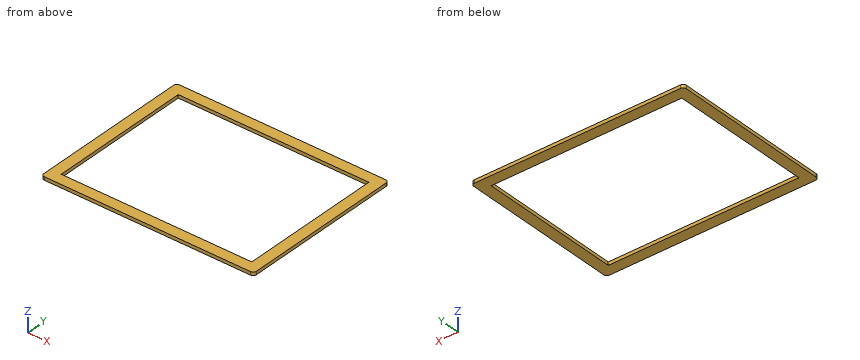
```python
from build123d import *

# Parameters (mm, degrees)
F0_W     = 194
F0_H     = 150
F1_DEPTH = 3
F2_W     = 174
F2_H     = 130
F3_DEPTH = 3
F4_R     = 3


with BuildPart() as f1:
    # F0 (on Top) → F1 (new body)
    with BuildSketch(Plane.XY):
        Rectangle(F0_W, F0_H)
    extrude(amount=F1_DEPTH)

    # F2 (on face) → F3 (cut, through all)
    with BuildSketch(Plane.XY.offset(3)):
        Rectangle(F2_W, F2_H)
    extrude(amount=-F3_DEPTH, mode=Mode.SUBTRACT)

    # F4
    f4_edges = [f1.edges().sort_by_distance(p)[0] for p in [
        (-97, -75, 1.5),
        (97, -75, 1.5),
        (97, 75, 1.5),
        (-97, 75, 1.5),
    ]]
    fillet(f4_edges, radius=F4_R)


solid = f1.part
```
Model file for the job. Use its own axes, mm. Coordinates: 2 decimals unless noted, no trailing zeros. Order: outer loops, then holes, each group sorted by start corner. A loop starts at its lowest first (then second) coordinate and runs counter-clockwise, first axis right, second up. Notation, with made-up numbers: M 40,-23.75 L 71,-23.75 A15 cw 71,-0.75 Z; hole C 85,-23 d8. An arc over 180 degrees is marked long. Answer as CSV lines item,"result".
(1) Band-saw the part on B-B, the plane z = 0.9. List the corners of the cut face in (x, y), then the cut area to 3 significant figures.
Geometry says:
outline,"M -97,-72 A3 ccw -94,-75 L 94,-75 A3 ccw 97,-72 L 97,72 A3 ccw 94,75 L -94,75 A3 ccw -97,72 Z; hole M -87,-65 L 87,-65 L 87,65 L -87,65 Z"
area,"6,470 mm2"
(2) Band-saw the part on C-C, the plane y = -29.5. List the corners of the cut face in (x, z).
Geometry says:
outline,"M -97,0 L -87,0 L -87,3 L -97,3 Z; M 87,0 L 97,0 L 97,3 L 87,3 Z"
(3) Band-saw the part on A-A, the plane x = -84.5. List the corners of the cut face in (y, z), then the cut area to 3 significant figures.
Geometry says:
outline,"M -75,0 L -65,0 L -65,3 L -75,3 Z; M 65,0 L 75,0 L 75,3 L 65,3 Z"
area,"60.0 mm2"
(4) Wall check: line 1 along X through (y, z) = (-26, 2.8); line 2 along Y through (x, z) = (72.5, 0.8). Give the ranges that are in metal, low to high.
Geometry says:
line 1,"x = -97 to -87, 87 to 97"
line 2,"y = -75 to -65, 65 to 75"
